CAD build for the part. Positions are in the model's coordinates, mm. A direction names the side the tool comes from. Give positions to 0.01 mm unless a question says otherwise; leave off trailing zeros. Order: outer loops, then holes, each group sorted by start corner. A loop starts at its lowest first (then second) coordinate and runs counter-clockwise, first axis right, second up.
```python
from build123d import *

# Parameters (mm, degrees)
SKETCH1_W           = 20
SKETCH1_H           = 20
BOSS_EXTRUDE1_DEPTH = 140
SKETCH2_R           = 5
CUT_EXTRUDE1_DEPTH  = 142.774468788
SKETCH3_W           = 10.2
SKETCH3_H           = 20
CUT_EXTRUDE2_DEPTH  = 142.774468788
FILLET1_R           = 5


with BuildPart() as part:
    # Sketch1 → Boss-Extrude1 (new body)
    with BuildSketch(Plane(origin=(0, 0, 0), x_dir=(1, 0, 0), z_dir=(0, 1, 0))):
        Rectangle(SKETCH1_W, SKETCH1_H)
    extrude(amount=BOSS_EXTRUDE1_DEPTH)

    # Sketch2 → Cut-Extrude1 (cut, through all)
    with BuildSketch(Plane.XY.offset(10)):
        with Locations((0, 10.125979961)):
            Circle(SKETCH2_R)
    extrude(amount=-CUT_EXTRUDE1_DEPTH, mode=Mode.SUBTRACT)

    # Sketch3 → Cut-Extrude2 (cut, through all)
    with BuildSketch(Plane(origin=(10, 0, 0), x_dir=(0, 0, -1), z_dir=(1, 0, 0))):
        with Locations((-0.09, 10)):
            Rectangle(SKETCH3_W, SKETCH3_H)
    extrude(amount=-CUT_EXTRUDE2_DEPTH, mode=Mode.SUBTRACT)

    # Fillet1
    # the kernel refuses this fillet: 5 mm, written as the material it takes off along each edge
    with BuildSketch(Plane(origin=(22.5, 0, -10), x_dir=(0, 0, 1), z_dir=(-1, 0, 0))) as fillet1_piece_1:
        with BuildLine():
            CenterArc((FILLET1_R, FILLET1_R), FILLET1_R, 180, 90)
            Line((0, FILLET1_R), (0, 0))
            Line((0, 0), (FILLET1_R, 0))
        make_face()
    extrude(amount=45, mode=Mode.SUBTRACT)
    with BuildSketch(Plane(origin=(-22.49097174, 0, 10), x_dir=(0, 1, 0), z_dir=(1, 0, 0))) as fillet1_piece_2:
        with BuildLine():
            CenterArc((4.996388696, -5), FILLET1_R, 90, 87.822236049)
            Line((0, -4.81), (0, 0))
            Line((0, 0), (4.996388696, 0))
        make_face()
    extrude(amount=44.981943479, mode=Mode.SUBTRACT)
    with BuildSketch(Plane(origin=(-10, -12.5, -10), x_dir=(0, 0, 1), z_dir=(0, 1, 0)), Plane(origin=(-10, -12.5, 10), x_dir=(1, 0, 0), z_dir=(0, 1, 0))) as fillet1_piece_3:
        with BuildLine():
            CenterArc((FILLET1_R, FILLET1_R), FILLET1_R, 180, 90)
            Line((0, FILLET1_R), (0, 0))
            Line((0, 0), (FILLET1_R, 0))
        make_face()
    extrude(amount=165, mode=Mode.SUBTRACT)
    with BuildSketch(Plane(origin=(10, -12.5, -10), x_dir=(0, 0, 1), z_dir=(0, 1, 0)), Plane(origin=(10, -12.5, 10), x_dir=(-1, 0, 0), z_dir=(0, 1, 0))) as fillet1_piece_4:
        with BuildLine():
            CenterArc((FILLET1_R, -FILLET1_R), FILLET1_R, 90, 90)
            Line((0, -FILLET1_R), (0, 0))
            Line((0, 0), (FILLET1_R, 0))
        make_face()
    extrude(amount=165, mode=Mode.SUBTRACT)


solid = part.part
```
Item 1: Two-plate mould, pull along Y, no slides. Class faces 3 (the face through (0, 20, 0)), 4 (the face through (-1.084, 5.245, 7.629)), 5 (the face through (8, 69, 9)): released by +Y, released by -Y, zero draft, split by the parting line, or undercut.
Item 2: Slice it at A-A (x = 0). Give the cut face in (y, z).
Item 3: Drop a flat-ended pin along its axis: pin 1 Ø1 at (x, y) = (7.5, 49.5) entering from +Z. Give the stop position or say it passes through.
Item 4: Tool access for faces 1 (the face through (2, 5, 5.19)), 2 (the face through (-9, 69, 8)): list every direction of +Z, -Z, +X, -X, +Y, -Y with a clear straight run to the whole face (end or side of a thin tool).
Item 5: Wall check: L1, parallel to Z at x = 3.5, y = 14.5; L2, parallel to Y at x = 7.75, z = 2.5; L3, parallel to Y at x = -1.5, z = 5.25. Give the ranges that are in metal, low to high.
Item 6: Slice it at D-D (x = -6.5). Give the cut face in (y, z).
Item 7: Slice it at B-B (y = 92.5). Give the cut face in (x, z).
Item 8: Slice it at C-C (z = -6.25). Give the cut face in (x, y).
A:
1. face 3: released by -Y
1. face 4: undercut
1. face 5: zero draft
2. outline: (0, -5.01) arc R5 ccw to (5, -10) - (5.13, -10) - (5.13, -5.01) - close; (0, 5.19) - (5.13, 5.19) - (5.13, 10) - (5, 10) arc R5 ccw to start; (15.13, -10) - (140, -10) - (140, 10) - (15.13, 10) - (15.13, 5.19) - (20, 5.19) - (20, -5.01) - (15.13, -5.01) - close
3. pin 1: stops at z = 9.58
4. face 1: +X, -X, -Y
4. face 2: +Z, -X, +Y, -Y
5. L1: z = -10 to -5.01, 5.19 to 10
5. L2: y = 20 to 140
5. L3: y = 0 to 5.36, 14.9 to 140
6. outline: (0, -5.01) arc R5 ccw to (3.5, -9.77) - (140, -9.77) - (140, 9.77) - (3.5, 9.77) arc R5 ccw to (0, 5.19) - (20, 5.19) - (20, -5.01) - close
7. outline: (-10, -5) arc R5 ccw to (-5, -10) - (5, -10) arc R5 ccw to (10, -5) - (10, 5) arc R5 ccw to (5, 10) - (-5, 10) arc R5 ccw to (-10, 5) - close
8. outline: (-9.84, 0.16) - (9.84, 0.16) - (9.84, 140) - (-9.84, 140) - close; hole circle Ø10 at (0, 10.13)
